Verification items for the finished model (mm, model axes). A direction names the side the tool comes from. Round coordinates to 2 decimals unless told otherwise and drop trailing zeros. Write each loop counter-clockwise with the first axis right and the second up, starting at its lowest first coordinate (ties: lowest second). Pieces come first, ordered by that corner, then holes. Notation, with made-up numbers: M 19,-23 L 74,-23 A16 cw 74,-14 Z; hole C 33,14.5 d5. An arc over 180 degrees is marked long. Answer in a Markdown table with one row per item. Add a question column.
1. Draft check along Z on faces 1 (the cylindrical face through (-13.79, 41.897, 48.028)), 2 (the cylindrical face through (-54.29, 140.97, 54.58)), 3 (the cylindrical face through (30.703, 1.972, -33.571)). Enter one of: pulls with the +Z half, pulls with the -Z half, needs draft (parallel to the pull), parting line crosses it, or undercut.
2. Sectioned sample at D-D on x = 0. Record the cut outline in (y, z), plus the area to 3 significant figures.
3. Sectioned sample at B-B on x = -15. Record the cut outline in (y, z).
4. Sectioned sample at A-A on z = -33.45. Record the cut outline in (x, y).
5. Material ranges on probe 1 along Z at (x, y) = (33.45, 3.15); probe 2 along Z at (x, y) = (35, 95), recorded low to high.
6. Sectioned sample at C-C on y = 79. Count the separate pieces of the cut face and the enclosed holes in it, plus the area to 3 significant figures.
7. Go/stop test with flat-tipped pins: pin 1 Ø6 at (x, z) = (35, 15) entering from +Y; pin 2 Ø1.5 at (y, z) = (63.5, -19.5) entering from -X; pin 3 Ø5 at (x, z) = (33.45, -33.45) entering from +Y; pin 4 Ø8 at (x, y) = (-32.5, 18.5) entering from -Z. Record where each tip stops, or that it passes through.
8. Set-up check for faces 4 (the flat face through (-1, 68, 50)), 5 (the flat face through (-50, 68, 1)), 6 (the cylindrical face through (48, 69, 49)), 7 (the cylindrical face through (48.028, 41.897, 13.79)), 8 (the cylindrical face through (-49, 68, -48)): record each of +Z, -Z, +X, -X, +Y, -Y from which the full face is reachable in a straight line by a thin tool's end or side.
```python
from build123d import *

# Parameters (mm, degrees)
SKETCH1_W           = 100
SKETCH1_H           = 100
SKETCH1_R           = 10
SKETCH1_R_2         = 2.75
BOSS_EXTRUDE1_DEPTH = 4
SKETCH2_W           = 100
SKETCH2_H           = 100
SKETCH2_W_2         = 92
SKETCH2_H_2         = 92
BOSS_EXTRUDE2_DEPTH = 135
FILLET1_R           = 5
BOSS_EXTRUDE3_DEPTH = 4
FILLET2_R           = 2
CUT_EXTRUDE1_REACH  = 112
SKETCH4_R           = 2.25
CUT_EXTRUDE2_REACH  = 112
SKETCH5_R           = 2.25


with BuildPart() as part:
    # Sketch1 → Boss-Extrude1 (new body)
    with BuildSketch(Plane(origin=(0, 0, 0), x_dir=(1, 0, 0), z_dir=(0, 1, 0))):
        Rectangle(SKETCH1_W, SKETCH1_H)
        Circle(SKETCH1_R, mode=Mode.SUBTRACT)
        with Locations((33.45, 33.45)):
            Circle(SKETCH1_R_2, mode=Mode.SUBTRACT)
        with Locations((33.45, -33.45)):
            Circle(SKETCH1_R_2, mode=Mode.SUBTRACT)
        with Locations((-33.45, -33.45)):
            Circle(SKETCH1_R_2, mode=Mode.SUBTRACT)
        with Locations((-33.45, 33.45)):
            Circle(SKETCH1_R_2, mode=Mode.SUBTRACT)
    extrude(amount=BOSS_EXTRUDE1_DEPTH)

    # Sketch2 → Boss-Extrude2 (add)
    with BuildSketch(Plane(origin=(0, 4, 0), x_dir=(1, 0, 0), z_dir=(0, 1, 0))):
        Rectangle(SKETCH2_W, SKETCH2_H)
        Rectangle(SKETCH2_W_2, SKETCH2_H_2, mode=Mode.SUBTRACT)
    extrude(amount=BOSS_EXTRUDE2_DEPTH)

    # Fillet1
    fillet1_edges = [part.edges().sort_by_distance(p)[0] for p in [
        (-46, 71.5, 46),
        (46, 71.5, 46),
        (46, 71.5, -46),
        (-46, 71.5, -46),
        (-50, 69.5, -50),
        (50, 69.5, -50),
        (50, 69.5, 50),
        (-50, 69.5, 50),
    ]]
    fillet(fillet1_edges, radius=FILLET1_R)

    # Sketch3 → Boss-Extrude3 (add)
    with BuildSketch(Plane(origin=(0, 139, 0), x_dir=(1, 0, 0), z_dir=(0, 1, 0))):
        with BuildLine():
            Line((-41, 60), (41, 60))
            ThreePointArc((41, 60), (54.435028843, 54.435028843), (60, 41))
            Line((60, 41), (60, -41))
            ThreePointArc((60, -41), (54.435028843, -54.435028843), (41, -60))
            Line((41, -60), (-41, -60))
            ThreePointArc((-41, -60), (-54.435028843, -54.435028843), (-60, -41))
            Line((-60, -41), (-60, 41))
            ThreePointArc((-60, 41), (-54.435028843, 54.435028843), (-41, 60))
        make_face()
        with BuildLine():
            Line((-41, 46), (41, 46))
            ThreePointArc((41, 46), (44.535533906, 44.535533906), (46, 41))
            Line((46, 41), (46, -41))
            ThreePointArc((46, -41), (44.535533906, -44.535533906), (41, -46))
            Line((41, -46), (-41, -46))
            ThreePointArc((-41, -46), (-44.535533906, -44.535533906), (-46, -41))
            Line((-46, -41), (-46, 41))
            ThreePointArc((-46, 41), (-44.535533906, 44.535533906), (-41, 46))
        make_face(mode=Mode.SUBTRACT)
    extrude(amount=BOSS_EXTRUDE3_DEPTH)

    # Fillet2
    fillet2_edges = [part.edges().sort_by_distance(p)[0] for p in [
        (0, 139, 50),
        (-50, 139, 0),
        (50, 139, 0),
        (0, 139, -50),
        (-48.535533906, 139, -48.535533906),
        (48.535533906, 139, -48.535533906),
        (48.535533906, 139, 48.535533906),
        (-48.535533906, 139, 48.535533906),
    ]]
    fillet(fillet2_edges, radius=FILLET2_R)

    # Sketch4 → Cut-Extrude1 (cut, up to next)
    with BuildSketch(Plane(origin=(50, 0, 0), x_dir=(0, 0, -1), z_dir=(1, 0, 0)), mode=Mode.PRIVATE) as cut_extrude1_sk1:
        with Locations((-15, 79)):
            Circle(SKETCH4_R)
    cut_extrude1_tool1 = extrude(cut_extrude1_sk1.sketch, amount=-CUT_EXTRUDE1_REACH, mode=Mode.PRIVATE) & part.part
    add(cut_extrude1_tool1.solids().sort_by_distance((50, 79, 15))[0], mode=Mode.SUBTRACT)
    # Sketch4 → Cut-Extrude1 (cut, up to next)
    with BuildSketch(Plane(origin=(50, 0, 0), x_dir=(0, 0, -1), z_dir=(1, 0, 0)), mode=Mode.PRIVATE) as cut_extrude1_sk2:
        with Locations((15, 79)):
            Circle(SKETCH4_R)
    cut_extrude1_tool2 = extrude(cut_extrude1_sk2.sketch, amount=-CUT_EXTRUDE1_REACH, mode=Mode.PRIVATE) & part.part
    add(cut_extrude1_tool2.solids().sort_by_distance((50, 79, -15))[0], mode=Mode.SUBTRACT)
    # Sketch4 → Cut-Extrude1 (cut, up to next)
    with BuildSketch(Plane(origin=(50, 0, 0), x_dir=(0, 0, -1), z_dir=(1, 0, 0)), mode=Mode.PRIVATE) as cut_extrude1_sk3:
        with Locations((15, 40)):
            Circle(SKETCH4_R)
    cut_extrude1_tool3 = extrude(cut_extrude1_sk3.sketch, amount=-CUT_EXTRUDE1_REACH, mode=Mode.PRIVATE) & part.part
    add(cut_extrude1_tool3.solids().sort_by_distance((50, 40, -15))[0], mode=Mode.SUBTRACT)
    # Sketch4 → Cut-Extrude1 (cut, up to next)
    with BuildSketch(Plane(origin=(50, 0, 0), x_dir=(0, 0, -1), z_dir=(1, 0, 0)), mode=Mode.PRIVATE) as cut_extrude1_sk4:
        with Locations((-15, 40)):
            Circle(SKETCH4_R)
    cut_extrude1_tool4 = extrude(cut_extrude1_sk4.sketch, amount=-CUT_EXTRUDE1_REACH, mode=Mode.PRIVATE) & part.part
    add(cut_extrude1_tool4.solids().sort_by_distance((50, 40, 15))[0], mode=Mode.SUBTRACT)

    # Sketch5 → Cut-Extrude2 (cut, up to next)
    with BuildSketch(Plane.XY.offset(50), mode=Mode.PRIVATE) as cut_extrude2_sk1:
        with Locations((15, 79)):
            Circle(SKETCH5_R)
    cut_extrude2_tool1 = extrude(cut_extrude2_sk1.sketch, amount=-CUT_EXTRUDE2_REACH, mode=Mode.PRIVATE) & part.part
    add(cut_extrude2_tool1.solids().sort_by_distance((15, 79, 50))[0], mode=Mode.SUBTRACT)
    # Sketch5 → Cut-Extrude2 (cut, up to next)
    with BuildSketch(Plane.XY.offset(50), mode=Mode.PRIVATE) as cut_extrude2_sk2:
        with Locations((-15, 79)):
            Circle(SKETCH5_R)
    cut_extrude2_tool2 = extrude(cut_extrude2_sk2.sketch, amount=-CUT_EXTRUDE2_REACH, mode=Mode.PRIVATE) & part.part
    add(cut_extrude2_tool2.solids().sort_by_distance((-15, 79, 50))[0], mode=Mode.SUBTRACT)
    # Sketch5 → Cut-Extrude2 (cut, up to next)
    with BuildSketch(Plane.XY.offset(50), mode=Mode.PRIVATE) as cut_extrude2_sk3:
        with Locations((-15, 40)):
            Circle(SKETCH5_R)
    cut_extrude2_tool3 = extrude(cut_extrude2_sk3.sketch, amount=-CUT_EXTRUDE2_REACH, mode=Mode.PRIVATE) & part.part
    add(cut_extrude2_tool3.solids().sort_by_distance((-15, 40, 50))[0], mode=Mode.SUBTRACT)
    # Sketch5 → Cut-Extrude2 (cut, up to next)
    with BuildSketch(Plane.XY.offset(50), mode=Mode.PRIVATE) as cut_extrude2_sk4:
        with Locations((15, 40)):
            Circle(SKETCH5_R)
    cut_extrude2_tool4 = extrude(cut_extrude2_sk4.sketch, amount=-CUT_EXTRUDE2_REACH, mode=Mode.PRIVATE) & part.part
    add(cut_extrude2_tool4.solids().sort_by_distance((15, 40, 50))[0], mode=Mode.SUBTRACT)


solid = part.part
```
Geometry check:
| question | item | result |
|---|---|---|
| 1 | face 1 | needs draft |
| 1 | face 2 | pulls with the +Z half |
| 1 | face 3 | undercut |
| 2 | outline | M 0,-50 L 137,-50 A2 cw 139,-52 L 139,-60 L 143,-60 L 143,-46 L 4,-46 L 4,-10 L 0,-10 Z; M 0,10 L 4,10 L 4,46 L 143,46 L 143,60 L 139,60 L 139,52 A2 cw 137,50 L 0,50 Z |
| 2 | area | 1,510 mm2 |
| 3 | outline | M 0,-50 L 137,-50 A2 cw 139,-52 L 139,-60 L 143,-60 L 143,-46 L 4,-46 L 4,46 L 37.75,46 L 37.75,50 L 0,50 Z; M 42.25,46 L 76.75,46 L 76.75,50 L 42.25,50 Z; M 81.25,46 L 143,46 L 143,60 L 139,60 L 139,52 A2 cw 137,50 L 81.25,50 Z |
| 4 | outline | M -60,139 L -52,139 A2 cw -50,137 L -50,0 L -36.2,0 L -36.2,4 L -46,4 L -46,143 L -60,143 Z; M -30.7,0 L 30.7,0 L 30.7,4 L -30.7,4 Z; M 36.2,0 L 50,0 L 50,137 A2 cw 52,139 L 60,139 L 60,143 L 46,143 L 46,4 L 36.2,4 Z |
| 5 | probe 1 | z = -50 to -36.2, -30.7 to 30.7, 36.2 to 50 |
| 5 | probe 2 | z = -50 to -46, 46 to 50 |
| 6 | separate pieces | 4 |
| 6 | enclosed holes | 0 |
| 6 | area | 1,460 mm2 |
| 7 | pin 1 | stops at y = 4 |
| 7 | pin 2 | stops at x = -50 |
| 7 | pin 3 | passes through |
| 7 | pin 4 | stops at z = -50 |
| 8 | face 4 | +Z, +X, -X, -Y |
| 8 | face 5 | +Z, -Z, -X, -Y |
| 8 | face 6 | +Z, +X, -Y |
| 8 | face 7 | +X |
| 8 | face 8 | -Z, -X, -Y |
